from build123d import *

# Parameters (mm, degrees)
SKETCH1_R                      = 31.75
BOSS_EXTRUDE1_DEPTH            = 33.3375
F_3_8_CLEARANCE_HOLE1_D        = 10.0838
SKETCH4_R                      = 21.082
CUT_EXTRUDE1_DEPTH             = 50.8
CUT_EXTRUDE1_DEPTH_BACK        = 50.8
TAP_DRILL_FOR_10_24_TAP1_D     = 3.7973
TAP_DRILL_FOR_10_24_TAP1_DEPTH = 19.05
TAP_DRILL_FOR_10_24_TAP1_TIP   = 1.140824014


with BuildPart() as part:
    # Sketch1 → Boss-Extrude1 (new body)
    with BuildSketch(Plane(origin=(0, 0, 0), x_dir=(1, 0, 0), z_dir=(0, 1, 0))):
        Circle(SKETCH1_R)
    extrude(amount=BOSS_EXTRUDE1_DEPTH)

    # 3_8 Clearance Hole1 (through all)
    with Locations(Plane(origin=(0, 33.3375, 0), x_dir=(1, 0, 0), z_dir=(0, 1, 0))):
        with Locations((0, 0)):
            Hole(F_3_8_CLEARANCE_HOLE1_D / 2)

    # Sketch4 → Cut-Extrude1 (cut, two sides)
    with BuildSketch(Plane.XY) as cut_extrude1_sk:
        with Locations((0, 33.3375)):
            Circle(SKETCH4_R)
    extrude(amount=CUT_EXTRUDE1_DEPTH, mode=Mode.SUBTRACT)
    extrude(cut_extrude1_sk.sketch, amount=-CUT_EXTRUDE1_DEPTH_BACK, mode=Mode.SUBTRACT)

    # Tap Drill for _10-24 Tap1
    with Locations(Plane(origin=(0, 0, 0), x_dir=(-1, 0, 0), z_dir=(0, -1, 0))):
        with Locations((25.4, -9.525), (25.4, 9.525), (-25.4, 9.525), (-25.4, -9.525)):
            Hole(TAP_DRILL_FOR_10_24_TAP1_D / 2, depth=TAP_DRILL_FOR_10_24_TAP1_DEPTH)
            with Locations((0, 0, -(TAP_DRILL_FOR_10_24_TAP1_DEPTH + TAP_DRILL_FOR_10_24_TAP1_TIP / 2))):  # 118° drill point
                Cone(0, TAP_DRILL_FOR_10_24_TAP1_D / 2, TAP_DRILL_FOR_10_24_TAP1_TIP, mode=Mode.SUBTRACT)


solid = part.part
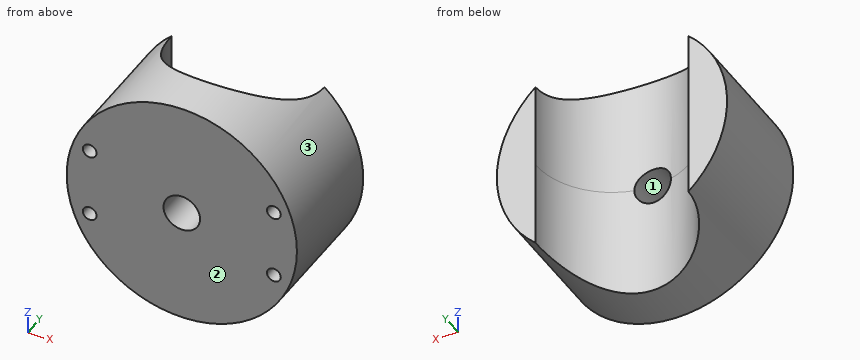
Geometry: final body of the model. Coordinates: model frame, mm. Face numbers are marked on the shaded views. Round coordinates to 2 decimals unless told otherwise and drop trailing zeros. Order: outer loops, then holes, each group sorted by start corner. A loop starts at its lowest first (then second) coordinate and runs counter-clockwise, first axis right, second up.
Q1. Section B-B, the plane y = 15. Output: boundary loops of the cut face in (x, z) (3 decimals).
Result sheet:
outline: (-10.401, -29.998) - (-10.401, 29.998) arc R31.75 ccw to start; (10.401, -29.998) arc R31.75 ccw to (10.401, 29.998) - close; hole circle Ø3.797 at (-25.4, -9.525); hole circle Ø3.797 at (-25.4, 9.525); hole circle Ø3.797 at (25.4, -9.525); hole circle Ø3.797 at (25.4, 9.525)
Q2. Pin query (flat end, axial travel): pin 1 (4 mm diameter, centred on x = -18, y = 15.5, fed in from +Z); pin 2 (1.5 mm diameter, centred on y = 16.5, z = -10, fed in from -X); pin 3 (6 mm diameter, centred on x = 0, z = 0, fed in from -Y); pin 4 (3 mm diameter, centred on x = -15, z = -6, fed in from +Y) (3 decimals). Return the tip coordinate at first contact, or that it passes through.
Result sheet:
pin 1: stops at z = 27.42
pin 2: stops at x = -30.37
pin 3: passes through
pin 4: stops at y = 20.215
Q3. Mould query, pull axis X, two halves, no side actions, for the marked faces 1, 2 and 3. Classes: released by +X, released by -X, zero draft, split by the parting line, or undercut.
Result sheet:
face 1: undercut
face 2: zero draft
face 3: split by the parting line
Q4. Section C-C, the plane z = -1. Output: boundary loops of the cut face in (x, y).
Result sheet:
outline: (-31.73, 0) - (-4.94, 0) - (-4.94, 12.84) arc R21.08 cw to (-21.08, 33.34) - (-31.73, 33.34) - close; (4.94, 0) - (31.73, 0) - (31.73, 33.34) - (21.08, 33.34) arc R21.08 cw to (4.94, 12.84) - close
Q5. Material intervals for probe 1 along X at (y, z) = (9.5, 8.5); probe 2 along Z at (x, y) = (-25, 12); probe 3 along Z at (x, y) = (0, 8.5), sorted ascending.
Result sheet:
probe 1: x = -30.59 to -27, -23.8 to 23.8, 27 to 30.59
probe 2: z = -19.57 to -11.38, -7.67 to 7.67, 11.38 to 19.57
probe 3: z = -31.75 to -5.04, 5.04 to 31.75
Q6. Section A-A, the plane x = 0. Output: boundary loops of the cut face in (y, z), and give its area (3 significant figures).
Result sheet:
outline: (0, -31.75) - (12.26, -31.75) - (12.26, -5.04) - (0, -5.04) - close; (0, 5.04) - (12.26, 5.04) - (12.26, 31.75) - (0, 31.75) - close
area: 655 mm2
Q7. Section D-D, the plane y = 11. Output: boundary loops of the cut face in (x, z) (3 decimals).
Result sheet:
outline: circle Ø63.5 at (0, 0); hole circle Ø3.797 at (-25.4, -9.525); hole circle Ø3.797 at (-25.4, 9.525); hole circle Ø10.084 at (0, 0); hole circle Ø3.797 at (25.4, -9.525); hole circle Ø3.797 at (25.4, 9.525)
